```python
from build123d import *
from build123d.topology import SkipClean

# Parameters (mm, degrees)
SKETCH_1_W                       = 400
SKETCH_1_H                       = 135
SKETCH_1_R                       = 3
SM_BASE_FLANGE_1_DEPTH           = 0.7
SM_EDGE_FLANGE_1_STRIP_W         = 3.2
SM_EDGE_FLANGE_1_STRIP_H         = 0.7
SM_EDGE_FLANGE_1_STRIP_CUT_DEPTH = 400
SM_EDGE_FLANGE_1_DEPTH           = 400
MOVE_START                       = -0.5
MOVE_BODY_1_OUTLINE_W            = 400
MOVE_BODY_1_OUTLINE_H            = 134.3
MOVE_BODY_1_OUTLINE_R            = 3
MOVE_BODY_1_DEPTH                = 0.5
MOVE_START_2                     = -4
MOVE_BODY_1_2_OUTLINE_W          = 400
MOVE_BODY_1_2_OUTLINE_H          = 0.7
MOVE_BODY_1_2_DEPTH              = 2.6
MOVE_START_3                     = -1.315058
MOVE_BODY_1_3_OUTLINE_W          = 400
MOVE_BODY_1_3_OUTLINE_H          = 134.3
MOVE_BODY_1_3_OUTLINE_R          = 3
MOVE_BODY_1_3_DEPTH              = 0.615058
MOVE_BODY_1_4_OUTLINE_W          = 400
MOVE_BODY_1_4_OUTLINE_H          = 0.7
MOVE_BODY_1_4_DEPTH              = 3.1
MOVE_START_4                     = -1.4
MOVE_BODY_1_5_OUTLINE_W          = 400
MOVE_BODY_1_5_OUTLINE_H          = 134.3
MOVE_BODY_1_5_OUTLINE_R          = 3
MOVE_BODY_1_5_DEPTH              = 0.084942
MOVE_START_5                     = -0.639415385
MOVE_BODY_1_6_OUTLINE_W          = 400
MOVE_BODY_1_6_OUTLINE_H          = 0.7
MOVE_BODY_1_6_DEPTH              = 0.139415385
MOVE_START_6                     = -200
MOVE_BODY_1_7_DEPTH              = 400
MOVE_BODY_1_8_DEPTH              = 400


with BuildPart() as part:
    # 基体-法兰1: sheet metal written as solids
    # 草图1 → 基体-法兰1 (new body)
    with BuildSketch(Plane(origin=(0, 0, 0), x_dir=(1, 0, 0), z_dir=(0, 1, 0))):
        Rectangle(SKETCH_1_W, SKETCH_1_H)
        with Locations(Location((-194.5, -60.5, 0), (0, 0, 270))):
            Circle(SKETCH_1_R, mode=Mode.SUBTRACT)
        with Locations(Location((-194.5, -10.5, 0), (0, 0, 270))):
            Circle(SKETCH_1_R, mode=Mode.SUBTRACT)
        with Locations(Location((-194.5, -0.5, 0), (0, 0, 270))):
            Circle(SKETCH_1_R, mode=Mode.SUBTRACT)
        with Locations(Location((-194.5, 49.5, 0), (0, 0, 270))):
            Circle(SKETCH_1_R, mode=Mode.SUBTRACT)
        with Locations(Location((0, -10.5, 0), (0, 0, 270))):
            Circle(SKETCH_1_R, mode=Mode.SUBTRACT)
        with Locations(Location((0, -0.5, 0), (0, 0, 270))):
            Circle(SKETCH_1_R, mode=Mode.SUBTRACT)
        with Locations(Location((194.5, -60.5, 0), (0, 0, 90))):
            Circle(SKETCH_1_R, mode=Mode.SUBTRACT)
        with Locations(Location((194.5, -10.5, 0), (0, 0, 90))):
            Circle(SKETCH_1_R, mode=Mode.SUBTRACT)
        with Locations(Location((194.5, -0.5, 0), (0, 0, 90))):
            Circle(SKETCH_1_R, mode=Mode.SUBTRACT)
        with Locations(Location((194.5, 49.5, 0), (0, 0, 90))):
            Circle(SKETCH_1_R, mode=Mode.SUBTRACT)
        with Locations(Location((174.5, 49.5, 0), (0, 0, 270))):
            Circle(SKETCH_1_R, mode=Mode.SUBTRACT)
    extrude(amount=-SM_BASE_FLANGE_1_DEPTH)

    # 边线-法兰1: sheet metal written as solids
    # 边线-法兰1 strip (on a plane across the edge) → 边线-法兰1 strip cut (cut)
    with BuildSketch(Plane(origin=(-200, -0.7, -67.5), x_dir=(0, 0, 1), z_dir=(1, 0, 0))):
        with Locations((-0.7, -0.35)):
            Rectangle(SM_EDGE_FLANGE_1_STRIP_W, SM_EDGE_FLANGE_1_STRIP_H)
    extrude(amount=SM_EDGE_FLANGE_1_STRIP_CUT_DEPTH, mode=Mode.SUBTRACT)

    # 边线-法兰1 section (on a plane across the edge) → 边线-法兰1 (add)
    with BuildSketch(Plane(origin=(-200, -0.7, -67.5), x_dir=(0, 0, 1), z_dir=(1, 0, 0))):
        with BuildLine():
            Line((0, 0.2), (0, 3.3))
            Line((0, 3.3), (0.7, 3.3))
            Line((0.7, 3.3), (0.7, 0.2))
            ThreePointArc((0.7, 0.2), (0.758578644, 0.058578644), (0.9, 0))
            Line((0.9, 0), (0.9, -0.7))
            ThreePointArc((0.9, -0.7), (0.263603897, -0.436396103), (0, 0.2))
        make_face()
    extrude(amount=SM_EDGE_FLANGE_1_DEPTH)

    # Move Body 1: read off the stored shape, not the designer's step
    # Move Body 1 outline → Move Body 1 (cut)
    with BuildSketch(Plane(origin=(0, 0, 0), x_dir=(1, 0, 0), z_dir=(0, 1, 0)).offset(MOVE_START)):
        with Locations((0, -0.35)):
            Rectangle(MOVE_BODY_1_OUTLINE_W, MOVE_BODY_1_OUTLINE_H)
        with Locations((-194.5, -60.5)):
            Circle(MOVE_BODY_1_OUTLINE_R, mode=Mode.SUBTRACT)
        with Locations((-194.5, -10.5)):
            Circle(MOVE_BODY_1_OUTLINE_R, mode=Mode.SUBTRACT)
        with Locations((-194.5, -0.5)):
            Circle(MOVE_BODY_1_OUTLINE_R, mode=Mode.SUBTRACT)
        with Locations((194.5, -60.5)):
            Circle(MOVE_BODY_1_OUTLINE_R, mode=Mode.SUBTRACT)
        with Locations((0, -10.5)):
            Circle(MOVE_BODY_1_OUTLINE_R, mode=Mode.SUBTRACT)
        with Locations((0, -0.5)):
            Circle(MOVE_BODY_1_OUTLINE_R, mode=Mode.SUBTRACT)
        with Locations((194.5, -10.5)):
            Circle(MOVE_BODY_1_OUTLINE_R, mode=Mode.SUBTRACT)
        with Locations((194.5, -0.5)):
            Circle(MOVE_BODY_1_OUTLINE_R, mode=Mode.SUBTRACT)
        with Locations((-194.5, 49.5)):
            Circle(MOVE_BODY_1_OUTLINE_R, mode=Mode.SUBTRACT)
        with Locations((174.5, 49.5)):
            Circle(MOVE_BODY_1_OUTLINE_R, mode=Mode.SUBTRACT)
        with Locations((194.5, 49.5)):
            Circle(MOVE_BODY_1_OUTLINE_R, mode=Mode.SUBTRACT)
    extrude(amount=MOVE_BODY_1_DEPTH, mode=Mode.SUBTRACT)

    # Move Body 1 2 outline → Move Body 1 2 (cut)
    with BuildSketch(Plane(origin=(0, 0, 0), x_dir=(1, 0, 0), z_dir=(0, 1, 0)).offset(MOVE_START_2)):
        with Locations((0, 67.15)):
            Rectangle(MOVE_BODY_1_2_OUTLINE_W, MOVE_BODY_1_2_OUTLINE_H)
    extrude(amount=MOVE_BODY_1_2_DEPTH, mode=Mode.SUBTRACT)

    # Move Body 1 3 outline → Move Body 1 3 (add)
    with SkipClean():  # the faces are left unmerged after this step: merging them gives an invalid solid
        with BuildSketch(Plane(origin=(0, 0, 0), x_dir=(1, 0, 0), z_dir=(0, 1, 0)).offset(MOVE_START_3)):
            with Locations((0, -0.35)):
                Rectangle(MOVE_BODY_1_3_OUTLINE_W, MOVE_BODY_1_3_OUTLINE_H)
            with Locations((-194.5, -60.5)):
                Circle(MOVE_BODY_1_3_OUTLINE_R, mode=Mode.SUBTRACT)
            with Locations((-194.5, -10.5)):
                Circle(MOVE_BODY_1_3_OUTLINE_R, mode=Mode.SUBTRACT)
            with Locations((-194.5, -0.5)):
                Circle(MOVE_BODY_1_3_OUTLINE_R, mode=Mode.SUBTRACT)
            with Locations((194.5, -60.5)):
                Circle(MOVE_BODY_1_3_OUTLINE_R, mode=Mode.SUBTRACT)
            with Locations((0, -10.5)):
                Circle(MOVE_BODY_1_3_OUTLINE_R, mode=Mode.SUBTRACT)
            with Locations((0, -0.5)):
                Circle(MOVE_BODY_1_3_OUTLINE_R, mode=Mode.SUBTRACT)
            with Locations((194.5, -10.5)):
                Circle(MOVE_BODY_1_3_OUTLINE_R, mode=Mode.SUBTRACT)
            with Locations((194.5, -0.5)):
                Circle(MOVE_BODY_1_3_OUTLINE_R, mode=Mode.SUBTRACT)
            with Locations((-194.5, 49.5)):
                Circle(MOVE_BODY_1_3_OUTLINE_R, mode=Mode.SUBTRACT)
            with Locations((174.5, 49.5)):
                Circle(MOVE_BODY_1_3_OUTLINE_R, mode=Mode.SUBTRACT)
            with Locations((194.5, 49.5)):
                Circle(MOVE_BODY_1_3_OUTLINE_R, mode=Mode.SUBTRACT)
        extrude(amount=MOVE_BODY_1_3_DEPTH)

    # Move Body 1 4 outline → Move Body 1 4 (add)
    with SkipClean():  # the faces are left unmerged after this step: merging them gives an invalid solid
        with BuildSketch(Plane(origin=(0, 0, 0), x_dir=(1, 0, 0), z_dir=(0, 1, 0)).offset(MOVE_START)):
            with Locations((0, 67.15)):
                Rectangle(MOVE_BODY_1_4_OUTLINE_W, MOVE_BODY_1_4_OUTLINE_H)
        extrude(amount=MOVE_BODY_1_4_DEPTH)

    # Move Body 1 5 outline → Move Body 1 5 (add)
    with SkipClean():  # the faces are left unmerged after this step: merging them gives an invalid solid
        with BuildSketch(Plane(origin=(0, 0, 0), x_dir=(1, 0, 0), z_dir=(0, 1, 0)).offset(MOVE_START_4)):
            with Locations((0, -0.35)):
                Rectangle(MOVE_BODY_1_5_OUTLINE_W, MOVE_BODY_1_5_OUTLINE_H)
            with Locations((-194.5, -60.5)):
                Circle(MOVE_BODY_1_5_OUTLINE_R, mode=Mode.SUBTRACT)
            with Locations((-194.5, -10.5)):
                Circle(MOVE_BODY_1_5_OUTLINE_R, mode=Mode.SUBTRACT)
            with Locations((-194.5, -0.5)):
                Circle(MOVE_BODY_1_5_OUTLINE_R, mode=Mode.SUBTRACT)
            with Locations((194.5, -60.5)):
                Circle(MOVE_BODY_1_5_OUTLINE_R, mode=Mode.SUBTRACT)
            with Locations((0, -10.5)):
                Circle(MOVE_BODY_1_5_OUTLINE_R, mode=Mode.SUBTRACT)
            with Locations((0, -0.5)):
                Circle(MOVE_BODY_1_5_OUTLINE_R, mode=Mode.SUBTRACT)
            with Locations((194.5, -10.5)):
                Circle(MOVE_BODY_1_5_OUTLINE_R, mode=Mode.SUBTRACT)
            with Locations((194.5, -0.5)):
                Circle(MOVE_BODY_1_5_OUTLINE_R, mode=Mode.SUBTRACT)
            with Locations((-194.5, 49.5)):
                Circle(MOVE_BODY_1_5_OUTLINE_R, mode=Mode.SUBTRACT)
            with Locations((174.5, 49.5)):
                Circle(MOVE_BODY_1_5_OUTLINE_R, mode=Mode.SUBTRACT)
            with Locations((194.5, 49.5)):
                Circle(MOVE_BODY_1_5_OUTLINE_R, mode=Mode.SUBTRACT)
        extrude(amount=MOVE_BODY_1_5_DEPTH)

    # Move Body 1 6 outline → Move Body 1 6 (add)
    with SkipClean():  # the faces are left unmerged after this step: merging them gives an invalid solid
        with BuildSketch(Plane(origin=(0, 0, 0), x_dir=(1, 0, 0), z_dir=(0, 1, 0)).offset(MOVE_START_5)):
            with Locations((0, 67.15)):
                Rectangle(MOVE_BODY_1_6_OUTLINE_W, MOVE_BODY_1_6_OUTLINE_H)
        extrude(amount=MOVE_BODY_1_6_DEPTH)

    # Move Body 1 7 outline → Move Body 1 7 (cut)
    with BuildSketch(Plane.YZ.offset(MOVE_START_6)):
        with BuildLine():
            Line((-0.5, 67.5), (-0.7, 67.5))
            Line((-0.7, 67.5), (-0.7, -66.6))
            ThreePointArc((-0.7, -66.6), (-0.641421356, -66.741421356), (-0.5, -66.8))
            Line((-0.5, -66.8), (-0.5, 67.5))
        make_face()
        with BuildLine():
            ThreePointArc((-0.5, -67.5), (-0.569919006, -67.497279963), (-0.639415385, -67.489136295))
            Line((-0.639415385, -67.489136295), (-0.639415385, -67.5))
            Line((-0.639415385, -67.5), (-0.5, -67.5))
        make_face()
        with BuildLine():
            ThreePointArc((-0.7, -67.477496439), (-1.203562364, -67.161248608), (-1.4, -66.6))
            Line((-1.4, -66.6), (-1.4, -67.5))
            Line((-1.4, -67.5), (-0.9, -67.5))
            ThreePointArc((-0.9, -67.5), (-0.799368978, -67.494356415), (-0.7, -67.477496439))
        make_face()
    extrude(amount=MOVE_BODY_1_7_DEPTH, mode=Mode.SUBTRACT)

    # Move Body 1 8 outline → Move Body 1 8 (add)
    with BuildSketch(Plane.YZ.offset(MOVE_START_6)):
        with BuildLine():
            ThreePointArc((-0.639415385, -67.461449742), (-0.669567969, -67.47000062), (-0.7, -67.477496439))
            ThreePointArc((-0.7, -67.477496439), (-0.669807457, -67.483835634), (-0.639415385, -67.489136295))
            Line((-0.639415385, -67.489136295), (-0.639415385, -67.461449742))
        make_face()
    extrude(amount=MOVE_BODY_1_8_DEPTH)


solid = part.part
```
Could you check a few things on this model? Use its own coordinates, in mm. A direction names the side the tool comes from. Give positions to 0.01 mm unless a question says otherwise; leave off trailing zeros. Write each loop counter-clockwise with the first axis right and the second up, starting at its lowest first coordinate (ties: lowest second). Pieces come first, ordered by that corner, then holes. Notation, with made-up numbers: (45, -19.5) -> (68, -19.5) arc R20 cw to (68, -7.5) -> close; hole circle Ø6 at (17, 63.25). An arc over 180 degrees is marked (long way). Write each question's results on one line, items separated by ' | '.
1. I need wall thicknesses on L1, parallel to Z at x = 194.5, y = -0.75; L2, parallel to X at y = -0.95, z = 11; L3, parallel to Z at x = -4.5, y = 1.6. Which ranges of each line are inside material? Lowest first, please.
Check sheet entries:
L1: z = -67.46 to -52.5, -46.5 to -2.5, 3.5 to 7.5, 13.5 to 57.5, 63.5 to 67.5 | L2: x = -200 to -197.46, -191.54 to -2.96, 2.96 to 191.54, 197.46 to 200 | L3: z = -67.5 to -66.8
2. I want a section at B-B, the plane z = 33. Write out the boundary of the cut face in (x, y), then the cut area to 3 significant figures.
Check sheet entries:
outline: (-200, -1.4) -> (200, -1.4) -> (200, -0.7) -> (-200, -0.7) -> close | area: 280 mm²
3. On a 3-axis mill with a long thin cutter (end or side, diameter ignored), from which of +Z, -Z, +X, -X, +Y, -Y can I reach the whole of each face in a straight line? I mean faces 1 (the flat face through (-3, -0.7, -14)), 2 (the flat face through (-3, -1.4, -15)). Say none if no direction works.
Check sheet entries:
face 1: +Z, +X, -X, +Y | face 2: +Z, -Z, +X, -X, -Y
4. I want a section at C-C, the plane y = 1.85. Write out the boundary of the cut face in (x, z).
Check sheet entries:
outline: (-200, -67.5) -> (200, -67.5) -> (200, -66.8) -> (-200, -66.8) -> close
5. I want a section at A-A, the plane x = -107.5. Write out the boundary of the cut face in (y, z).
Check sheet entries:
outline: (-1.4, -66.6) arc R0.9 ccw to (-0.5, -67.5) -> (2.6, -67.5) -> (2.6, -66.8) -> (-0.5, -66.8) arc R0.2 cw to (-0.7, -66.6) -> (-0.7, 67.5) -> (-1.4, 67.5) -> close
6. Will these pins go through, and if not, where does the flat tip stop? pin 1 Ø5 at (x, z) = (194.5, 0.5) entering from -Y; pin 2 Ø2 at (x, z) = (155.5, -48) entering from +Y.
Check sheet entries:
pin 1: passes through | pin 2: stops at y = -0.7
